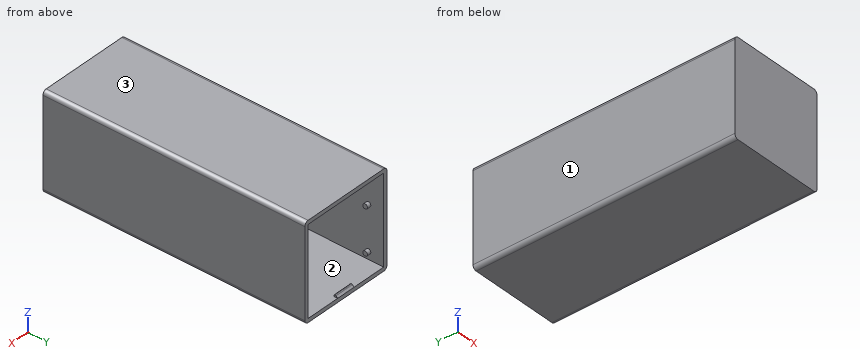
Autodesk Inventor part; units mm, degrees
ref_plane "YZ Plane" through (0, 0, 0) normal (1, 0, 0) x (0, 1, 0)
ref_plane "XZ Plane" through (0, 0, 0) normal (0, 1, 0) x (-1, 0, 0)
ref_plane "XY Plane" through (0, 0, 0) normal (0, 0, 1) x (1, 0, 0)
sketch "Sketch1" plane through (0, 0, 0) normal (0, 1, 0) x (-1, 0, 0)
  line L0 (0, 0) -> (50, 0)
  line L1 (50, 0) -> (50, -50)
  line L2 (50, -50) -> (0, -50)
  line L3 (0, -50) -> (0, 0)
  dimension "d0" = 50
  dimension "d1" = 50
extrude "Extrusion1" add sketch "Sketch1" along normal blind 2
sketch "Sketch2" plane through (0, 2, 0) normal (0, 1, 0) x (1, 0, 0)
  line L0 (-48, 2) -> (-2, 2)
  line L1 (-2, 2) -> (-2, 48)
  line L2 (-2, 48) -> (-48, 48)
  line L3 (-48, 48) -> (-48, 2)
  line L4 (0, 50) -> (-50, 50)
  line L5 (-50, 50) -> (-50, 0)
  line L6 (-50, 0) -> (0, 0)
  line L7 (0, 0) -> (0, 50)
  dimension "d4" = 2
  dimension "d5" = 2
  dimension "d6" = 2
  dimension "d7" = 2
extrude "Extrusion2" add sketch "Sketch2" along normal blind 135
fillet "Fillet1" radius 2 4 edges at (0, 68.5, 0) (0, 68.5, -50) (-50, 68.5, -50) (-50, 68.5, 0)
sketch "Sketch3" plane through (-2, 2, -48) normal (-1, 0, 0) x (0, 0, 1)
  circle A0 centre (4, 127) radius 1.25
  line L0 (0, 135) -> (46, 135)
  line L1 (0, -2) -> (0, 135)
  circle A1 centre (4, 94.5) radius 1.25
  circle A2 centre (24, 127) radius 1.25
  circle A3 centre (24, 94.5) radius 1.25
  point P0 (48, -2)
  dimension "d11" = 2.5
  dimension "d14" = 8
  dimension "d15" = 4
  dimension "d16" = 2.5
  dimension "d17" = 32.5
  dimension "d18" = 2.5
  dimension "d19" = 20
  dimension "d20" = 2.5
  dimension "d23" = 32.5
  dimension "d24" = 8
  dimension "d25" = 20
extrude "Extrusion3" add sketch "Sketch3" along normal blind 2
sketch "Sketch4" plane through (-48, 2, -2) normal (1, 0, 0) x (0, 0, -1)
  circle A0 centre (42, 127) radius 1.25
  line L0 (0, 135) -> (46, 135)
  line L1 (46, 135) -> (46, -2)
  circle A1 centre (42, 69) radius 1.25
  circle A2 centre (19, 127) radius 1.25
  circle A3 centre (19, 69) radius 1.25
  point P0 (-2, -2)
  dimension "d26" = 2.5
  dimension "d27" = 8
  dimension "d28" = 4
  dimension "d29" = 2.5
  dimension "d30" = 4
  dimension "d31" = 58
  dimension "d32" = 2.5
  dimension "d33" = 8
  dimension "d34" = 23
  dimension "d35" = 2.5
  dimension "d36" = 58
  dimension "d37" = 23
extrude "Extrusion4" add sketch "Sketch4" along normal blind 2
sketch "Sketch5" plane through (-48, 2, -48) normal (0, 0, 1) x (1, 0, 0)
  line L0 (46, 135) -> (0, 135) construction
  line L1 (46, 0) -> (46, 135)
  line L2 (0, 135) -> (46, 135)
  line L3 (23, 135) -> (23, 133) construction
  line L4 (23, 133) -> (28, 133)
  line L5 (23, 133) -> (18, 133)
  line L6 (18, 133) -> (24.2185, 133)
  line L7 (18, 133) -> (18, 135)
  line L8 (28, 133) -> (28, 135)
  point P0 (48, -2)
  dimension "d40" = 2
  dimension "d41" = 5
  dimension "d51" = 5
extrude "Extrusion5" add sketch "Sketch5" along normal blind 1
chamfer "Chamfer1" distance 1 angle 45 1 edges at (-25, 137, -47)
ref_plane "Work Plane1" through (-2, 137, -25) normal (0, 0, 1) x (1, 0, 0)
mirror "Mirror1" about plane through (-2, 137, -25) normal (0, 0, 1) of "Extrusion5"
chamfer "Chamfer2" distance 1 angle 45 1 edges at (-25, 137, -3)
fillet "Fillet2" radius 0.5 4 edges at (-25, 136, -47) (-25, 135, -47) (-25, 135, -3) (-25, 136, -3)
properties part number "180caseMain"
Design review of the part built by this model. Coordinates are the model's own, in mm. Face numbers are marked on the shaded views. Round coordinates to 2 decimals unless told otherwise and drop trailing zeros. Order: outer loops, then holes, each group sorted by start corner. A loop starts at its lowest first (then second) coordinate and runs counter-clockwise, first axis right, second up.
1) Clearance check with a flat-ended pin moving along its axis: pin 1 Ø2 at (x, z) = (-22, -28) entering from +Y. State where the tip first meets the part, or that it passes through.
The answers:
pin 1: stops at y = 2
2) Consider section C-C (z = -32). State the section outline as (x, y) points.
The answers:
outline: (-50, 0) - (0, 0) - (0, 137) - (-2, 137) - (-2, 2) - (-48, 2) - (-48, 137) - (-50, 137) - close
3) Consider section D-D (y = 96.5). State the section outline as (x, z) points, plus the area to 3 significant figures.
The answers:
outline: (-50, -48) arc R2 ccw to (-48, -50) - (-2, -50) arc R2 ccw to (0, -48) - (0, -2) arc R2 ccw to (-2, 0) - (-48, 0) arc R2 ccw to (-50, -2) - close; hole (-48, -48) - (-2, -48) - (-2, -45.25) - (-4, -45.25) - (-4, -42.75) - (-2, -42.75) - (-2, -25.25) - (-4, -25.25) - (-4, -22.75) - (-2, -22.75) - (-2, -2) - (-48, -2) - close
area: 391 mm2
4) For L1, parallel to Z at x = -44, y = 125.5; L2, parallel to Y at x = -37, z = -31, list the stretches that pass through material, from the lowest coordinate up.
The answers:
L1: z = -50 to -48, -2 to 0
L2: y = 0 to 2
5) Consider section A-A (y = 35). State the section outline as (x, z) points, plus the area to 3 significant figures.
The answers:
outline: (-50, -48) arc R2 ccw to (-48, -50) - (-2, -50) arc R2 ccw to (0, -48) - (0, -2) arc R2 ccw to (-2, 0) - (-48, 0) arc R2 ccw to (-50, -2) - close; hole (-48, -48) - (-2, -48) - (-2, -2) - (-48, -2) - close
area: 381 mm2
6) Draft analysis for pull direction X (two halves, no side actions). For the marked faces 1, 2 and 3, state which applies: released by +X, released by -X, zero draft, split by the parting line, or undercut.
The answers:
face 1: released by -X
face 2: undercut
face 3: zero draft
7) Consider section B-B (x = -11). State the section outline as (y, z) points.
The answers:
outline: (0, -50) - (137, -50) - (137, -48) - (2, -48) - (2, -2) - (137, -2) - (137, 0) - (0, 0) - close
